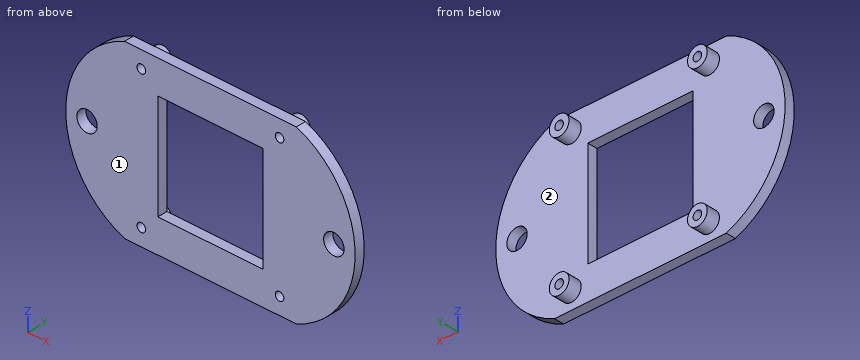
Autodesk Inventor part; units mm, degrees
ref_plane "YZ Plane" through (0, 0, 0) normal (1, 0, 0) x (0, 1, 0)
ref_plane "XZ Plane" through (0, 0, 0) normal (0, 1, 0) x (-1, 0, 0)
ref_plane "XY Plane" through (0, 0, 0) normal (0, 0, 1) x (1, 0, 0)
sketch "Sketch1" plane through (0, 0, 0) normal (0, 1, 0) x (-1, 0, 0)
  line L0 (0, 0) -> (52.2, 0)
  line L1 (52.2, 0) -> (52.2, -52.2)
  line L2 (52.2, -52.2) -> (0, -52.2)
  line L3 (0, -52.2) -> (0, 0)
  circle A0 centre (47.1, -47.1) radius 1.3
  circle A1 centre (5.1, -5.1) radius 1.3
  circle A2 centre (5.1, -47.1) radius 1.3
  line L4 (0, 0) -> (52.2, -52.2) construction
  line L5 (52.2, 0) -> (0, -52.2) construction
  line L6 (5.1, -5.1) -> (47.1, -47.1) construction
  circle A3 centre (47.1, -5.1) radius 1.3
  circle A4 centre (63.6, -26.1) radius 3.1
  circle A5 centre (-11.4, -26.1) radius 3.1
  arc A6 (52.2, -52.2) -> (52.2, 0) centre (42.0615, -26.1) ccw
  arc A7 (0, 0) -> (0, -52.2) centre (10.1385, -26.1) ccw
  line L7 (10.1, -10.1) -> (10.1, -42.1)
  line L8 (10.1, -42.1) -> (42.1, -42.1)
  line L9 (42.1, -42.1) -> (42.1, -10.1)
  line L10 (42.1, -10.1) -> (10.1, -10.1)
  line L11 (10.1, -10.1) -> (42.1, -42.1) construction
  line L12 (10.1, -42.1) -> (42.1, -10.1) construction
  point P0 (26.1, -26.1)
  point P1 (26.1, -26.1)
  dimension "d1" = 42
  dimension "d2" = 42
  dimension "d3" = 2.6
  dimension "d4" = 2.6
  dimension "d5" = 2.6
  dimension "d18" = 52.2
  dimension "d19" = 52.2
  dimension "d24" = 2.6
  dimension "d26" = 6.2
  dimension "d27" = 6.2
  dimension "d28" = 75
  dimension "d29" = 37.5
  dimension "d30" = 28
  dimension "d31" = 28
  dimension "d32" = 32
  dimension "d33" = 32
extrude "Extrusion1" add sketch "Sketch1" along normal blind 3
sketch "Sketch2" plane through (0, 3, 0) normal (0, 1, 0) x (1, 0, 0)
  circle A0 centre (-5.1, 5.1) radius 1.3
  circle A1 centre (-5.1, 5.1) radius 3
  circle A2 centre (-5.1, 47.1) radius 1.3
  circle A3 centre (-5.1, 47.1) radius 3
  circle A4 centre (-47.1, 47.1) radius 1.3
  circle A5 centre (-47.1, 47.1) radius 3
  circle A6 centre (-47.1, 5.1) radius 1.3
  circle A7 centre (-47.1, 5.1) radius 3
  point P0 (0, 0)
  dimension "d12" = 6
  dimension "d13" = 6
  dimension "d14" = 6
  dimension "d25" = 6
extrude "Extrusion2" add sketch "Sketch2" along normal blind 4
equation "\"d4\" = d3"
equation "\"d5\" = d3"
equation "\"d19\" = d18"
equation "\"d24\" = d3"
equation "\"d27\" = d26"
equation "\"d33\" = d32"
equation "\"d13\" = d12"
equation "\"d14\" = d12"
equation "\"d25\" = d12"
equation "\"d7\" = d8"
properties part number "ephys_board_rack"
Geometry: final body of the model. Coordinates: model frame, mm. Face numbers are marked on the shaded views. Round coordinates to 2 decimals unless told otherwise and drop trailing zeros. Order: outer loops, then holes, each group sorted by start corner. A loop starts at its lowest first (then second) coordinate and runs counter-clockwise, first axis right, second up.
Q1. Section C-C, the plane z = -12. Output: boundary loops of the cut face in (x, y).
Result sheet:
outline: (-66.25, 0) - (-42.1, 0) - (-42.1, 3) - (-66.25, 3) - close; (-10.1, 0) - (14.05, 0) - (14.05, 3) - (-10.1, 3) - close
Q2. Mould query, pull axis X, two halves, no side actions, for the marked faces 1 and 2. Classes: released by +X, released by -X, zero draft, split by the parting line, or undercut.
Result sheet:
face 1: zero draft
face 2: undercut
Q3. Material intervals for probe 1 along Z at (x, y) = (-47.1, 4); probe 2 along Z at (x, y) = (-47.1, 2.5), sorted ascending.
Result sheet:
probe 1: z = -50.1 to -48.4, -45.8 to -44.1, -8.1 to -6.4, -3.8 to -2.1
probe 2: z = -52.2 to -48.4, -45.8 to -6.4, -3.8 to 0
Q4. Section B-B, the plane x = -40. Output: boundary loops of the cut face in (y, z).
Result sheet:
outline: (0, -52.2) - (3, -52.2) - (3, -42.1) - (0, -42.1) - close; (0, -10.1) - (3, -10.1) - (3, 0) - (0, 0) - close
Q5. Section A-A, the plane y = 4. Output: boundary loops of the cut face in (x, z).
Result sheet:
outline: circle Ø6 at (-47.1, -47.1); circle Ø6 at (-47.1, -5.1); circle Ø6 at (-5.1, -47.1); circle Ø6 at (-5.1, -5.1); hole circle Ø2.6 at (-47.1, -47.1); hole circle Ø2.6 at (-47.1, -5.1); hole circle Ø2.6 at (-5.1, -47.1); hole circle Ø2.6 at (-5.1, -5.1)
Q6. Pin query (flat end, axial travel): pin 1 (3 mm diameter, centred on x = -5.1, z = -47.1, fed in from +Y); pin 2 (0.9 mm diameter, centred on y = 2, z = -28.5, fed in from -X); pin 3 (3.5 mm diameter, centred on y = 1.5, z = -19, fed in from +X); pin 4 (6 mm diameter, centred on x = -41, z = -46.5, fed in from +Y). Return the tip coordinate at first contact, or that it passes through.
Result sheet:
pin 1: stops at y = 7
pin 2: stops at x = -69.99
pin 3: stops at x = 17.35
pin 4: stops at y = 3
